Read the model definition and answer for the solid it produces. Units are mm, in the model's axes. Face numbers are marked on the shaded views. A direction names the side the tool comes from. Coordinates: 2 decimals unless noted, no trailing zeros. Order: outer loops, then holes, each group sorted by start corner. A loop starts at its lowest first (then second) coordinate and runs counter-clockwise, first axis right, second up. Notation, with made-up numbers: M -10,13.25 L 17,13.25 A15 ccw 17,33.25 Z; hole C 31.25,-22.5 d8. An arc over 180 degrees is marked long. Put each result on its own line as item: value.
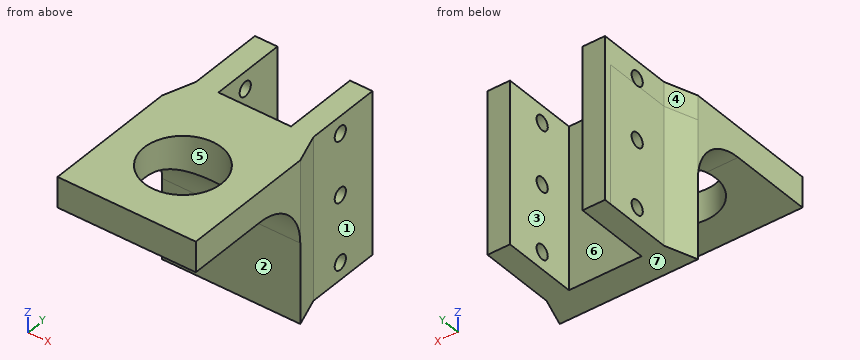
Autodesk Inventor part; units mm, degrees
ref_plane "YZ Plane" through (0, 0, 0) normal (1, 0, 0) x (0, 1, 0)
ref_plane "XZ Plane" through (0, 0, 0) normal (0, 1, 0) x (-1, 0, 0)
ref_plane "XY Plane" through (0, 0, 0) normal (0, 0, 1) x (1, 0, 0)
sketch "Sketch1" plane through (0, 0, 0) normal (0, 0, 1) x (1, 0, 0)
  line L0 (-25.4, -35.56) -> (25.4, -35.56)
  line L1 (25.4, -35.56) -> (25.4, 13.97)
  line L2 (25.4, 13.97) -> (-25.4, 13.97)
  line L3 (-25.4, 13.97) -> (-25.4, -35.56)
  line L4 (-25.4, -35.56) -> (25.4, 13.97) construction
  line L5 (25.4, -35.56) -> (-25.4, 13.97) construction
  line L6 (0, 25.146) -> (-12.7, 25.146)
  line L7 (-12.7, 25.146) -> (12.7, 25.146)
  line L8 (-12.7, 25.146) -> (-25.4, 13.97)
  line L9 (12.7, 25.146) -> (25.4, 13.97)
  line L10 (-12.7, 25.146) -> (-21.59, 25.146)
  line L11 (-21.59, 25.146) -> (-21.59, 50.546)
  line L12 (-21.59, 50.546) -> (-12.7, 50.546)
  line L13 (-12.7, 50.546) -> (-12.7, 25.146)
  line L14 (-21.59, 25.146) -> (-25.4, 13.97)
  line L15 (12.7, 25.146) -> (12.7, 50.546)
  line L16 (12.7, 50.546) -> (21.59, 50.546)
  line L17 (21.59, 50.546) -> (21.59, 25.146)
  line L18 (21.59, 25.146) -> (25.4, 13.97)
  line L19 (12.7, 25.146) -> (21.59, 25.146)
  circle A0 centre (0, -8.89) radius 14.224
  point P0 (0, 0)
  dimension "d1" = 49.53
  dimension "d2" = 50.8
  dimension "d6" = 8.89
  dimension "d7" = 25.4
  dimension "d8" = 8.89
  dimension "d47" = 11.176
  dimension "d51" = 28.448
  dimension "d52" = 34.036
  dimension "d53" = 43.18
extrude "Extrusion1" add sketch "Sketch1" along normal blind 8.89
sketch "Sketch3" plane through (0, 0, 0) normal (0, 0, -1) x (-1, 0, 0)
  circle A0 centre (0, 0) radius 14.224
  line L0 (21.5903, 3.302) -> (-21.59, 3.302)
  line L1 (-21.59, 3.302) -> (-21.59, 25.146)
  line L2 (-21.59, 25.146) -> (21.5903, 25.146)
  line L3 (21.5903, 25.146) -> (21.5903, 3.302)
  circle A1 centre (0, 0) radius 14.224
  line L4 (21.5903, 3.302) -> (-21.59, 25.146) construction
  line L5 (-21.59, 3.302) -> (21.5903, 25.146) construction
  line L6 (-25.4, -35.56) -> (-25.4, 13.97)
  line L7 (25.4, 13.97) -> (25.4, -35.56)
  line L8 (25.4, -35.56) -> (-25.4, -35.56)
  line L9 (25.4, 13.97) -> (25.4, -35.56)
  line L10 (21.59, 25.146) -> (25.4, 13.97)
  line L11 (21.59, 50.546) -> (21.59, 25.146)
  line L12 (12.7, 50.546) -> (21.59, 50.546)
  line L13 (12.7, 25.146) -> (12.7, 50.546)
  line L14 (-12.7, 25.146) -> (12.7, 25.146)
  line L15 (-12.7, 50.546) -> (-12.7, 25.146)
  line L16 (-21.59, 50.546) -> (-12.7, 50.546)
  line L17 (-21.59, 25.146) -> (-21.59, 50.546)
  line L18 (-25.4, 13.97) -> (-21.59, 25.146)
  line L19 (-25.4, -35.56) -> (-25.4, 13.97)
  line L20 (25.4, 3.302) -> (21.5903, 3.302)
  line L21 (-25.4, 3.302) -> (-21.59, 3.302)
  line L22 (0, 14.224) -> (-25.4, 14.224)
  point P0 (0.0002, 14.224)
  point P1 (-25.4, 13.97)
  point P2 (-13.8354, 3.302)
  point P3 (13.8354, 3.302)
  dimension "d13" = 28.448
extrude "Extrusion3" add sketch "Sketch3" along normal blind 50.8 contours A0 L22 L1 L2 L3 L0 | L0 L1 L22 A0 | L3 L10 L7 L20 | L21 L6 L18 L22 L1 | L22 L18 L1 | L2 L13 L12 L11 | L17 L16 L15 L2
sketch "Sketch5" plane through (21.59, 50.546, 8.89) normal (1, 0, 0) x (0, 0, -1)
  line L0 (59.69, -25.4) -> (59.69, 0)
  line L1 (0, -23.5788) -> (57.5469, -23.5788)
  line L2 (57.5469, 0) -> (57.5469, -23.5788)
  line L3 (59.69, 0) -> (59.69, -25.4)
  line L4 (59.69, 0) -> (0, 0)
  line L5 (0, -25.4) -> (0, 0)
  line L6 (59.69, -25.4) -> (0, -25.4)
  line L7 (0, -25.4) -> (0, -12.7)
  line L8 (0, -12.7) -> (57.5469, -12.7)
  circle A0 centre (6.35, -12.7) radius 2.6543
  circle A1 centre (53.34, -12.7) radius 2.6543
  circle A2 centre (28.7734, -12.7) radius 2.6543
  point P0 (8.89, -50.546)
  point P1 (59.69, -25.4)
  point P2 (31.4277, -12.7)
  point P3 (26.1191, -12.7)
  point P4 (55.9943, -12.7)
  point P5 (50.6857, -12.7)
  point P6 (9.0043, -12.7)
  point P7 (3.6957, -12.7)
  dimension "d39" = 12.7
  dimension "d40" = 5.3086
  dimension "d41" = 6.35
  dimension "d42" = 5.3086
  dimension "d43" = 6.35
  dimension "d44" = 5.3086
  dimension "d46" = 0
extrude "Extrusion4" cut sketch "Sketch5" against normal up to surface (43.18 mm away) contours A1 L8 | L8 A1 | A0 L8 | L8 A0 | A2 L8 | L8 A2
sketch "Sketch9" plane through (0, 0, -50.8) normal (0, 0, -1) x (-1, 0, 0)
  line L0 (-21.59, 50.546) -> (-12.7, 50.546)
  line L1 (13.335, -0.254) -> (-13.335, -0.254)
  line L2 (-13.335, -0.254) -> (-13.335, 50.546)
  line L3 (-13.335, 50.546) -> (13.335, 50.546)
  line L4 (13.335, 50.546) -> (13.335, -0.254)
  line L5 (-12.7, 25.146) -> (12.7, 25.146)
  line L6 (13.335, -0.254) -> (-13.335, 50.546) construction
  line L7 (-13.335, -0.254) -> (13.335, 50.546) construction
  line L8 (-25.4, -35.56) -> (-25.4, 13.97)
  line L9 (25.4, -13.97) -> (-25.4, -13.97)
  line L10 (-25.4, -13.97) -> (-25.4, 13.97)
  line L11 (-25.4, 13.97) -> (25.4, 13.97)
  line L12 (25.4, 13.97) -> (25.4, -13.97)
  line L13 (25.4, -13.97) -> (-25.4, 13.97) construction
  line L14 (-25.4, -13.97) -> (25.4, 13.97) construction
  point P0 (0, 0)
  point P1 (0, 25.146)
  point P2 (-13.335, 13.97)
  point P3 (13.335, 13.97)
  point P4 (-12.7, 50.546)
  dimension "d27" = 26.67
extrude "Extrusion5" cut sketch "Sketch9" against normal blind 42.8625
sketch "Sketch11" plane through (0, 0, 0) normal (0, 0, -1) x (-1, 0, 0)
  line L0 (25.4, 3.302) -> (13.8354, 3.302)
  line L1 (-13.8354, 3.302) -> (-25.4, 3.302)
  line L2 (-25.4, -35.56) -> (-25.4, 3.302)
  line L3 (25.4, -35.56) -> (-25.4, -35.56)
  line L4 (25.4, 3.302) -> (25.4, -35.56)
  line L5 (12.7, 25.146) -> (12.7, 50.546)
  line L6 (-12.7, 25.146) -> (12.7, 25.146)
  line L7 (-12.7, 50.546) -> (-12.7, 25.146)
  line L8 (-13.335, 50.546) -> (-12.7, 50.546)
  line L9 (-13.335, 13.97) -> (-13.335, 50.546)
  line L10 (-25.4, 13.97) -> (-13.335, 13.97)
  line L11 (-25.4, 3.302) -> (-25.4, 13.97)
  line L12 (-13.8354, 3.302) -> (-25.4, 3.302)
  arc A0 (13.8354, 3.302) -> (-13.8354, 3.302) centre (0, 0) ccw
  line L13 (25.4, 3.302) -> (13.8354, 3.302)
  line L14 (25.4, 13.97) -> (25.4, 3.302)
  line L15 (13.335, 13.97) -> (25.4, 13.97)
  line L16 (13.335, 50.546) -> (13.335, 13.97)
  line L17 (12.7, 50.546) -> (13.335, 50.546)
  arc A1 (13.8354, 3.302) -> (-13.8354, 3.302) centre (0, 0) ccw
extrude "Extrusion6" add sketch "Sketch11" along normal blind 2.286 contours L4 L3 L2 L1 A0 L0
sketch "Sketch12" plane through (0, 0, -7.9375) normal (0, 0, -1) x (-1, 0, 0)
  line L0 (12.7, 25.146) -> (12.7, 50.546)
  line L1 (-12.7, 25.146) -> (12.7, 25.146)
  line L2 (-12.7, 50.546) -> (-12.7, 25.146)
  line L3 (-13.335, 50.546) -> (-12.7, 50.546)
  line L4 (-13.335, 13.97) -> (-13.335, 50.546)
  line L5 (-25.4, 13.97) -> (-13.335, 13.97)
  line L6 (-25.4, 3.302) -> (-25.4, 13.97)
  line L7 (-13.8354, 3.302) -> (-25.4, 3.302)
  arc A0 (13.8354, 3.302) -> (-13.8354, 3.302) centre (0, 0) ccw
  line L8 (25.4, 3.302) -> (13.8354, 3.302)
  line L9 (25.4, 13.97) -> (25.4, 3.302)
  line L10 (13.335, 13.97) -> (25.4, 13.97)
  line L11 (13.335, 50.546) -> (13.335, 13.97)
  line L12 (12.7, 50.546) -> (13.335, 50.546)
extrude "Extrusion7" cut sketch "Sketch12" against normal blind 5.6515
sketch "Sketch13" plane through (0, 0, -2.286) normal (0, 0, -1) x (-1, 0, 0)
  line L0 (-12.7, 25.146) -> (12.7, 25.146)
  line L1 (-13.335, 13.97) -> (-13.335, 50.546)
  line L2 (12.7, 25.146) -> (-13.335, 25.146)
  line L3 (-13.335, 25.146) -> (-13.335, 50.546)
  line L4 (-13.335, 50.546) -> (12.7, 50.546)
  line L5 (12.7, 50.546) -> (12.7, 25.146)
  line L6 (13.335, 50.546) -> (13.335, 13.97)
  line L7 (12.7, 50.546) -> (13.335, 50.546)
  line L8 (13.335, 50.546) -> (13.335, 25.146)
  line L9 (13.335, 25.146) -> (12.7, 25.146)
  line L10 (12.7, 25.146) -> (12.7, 50.546)
  point P0 (0, 0)
  point P1 (-13.335, 25.146)
extrude "Extrusion8" cut sketch "Sketch13" against normal blind 37.211
sketch "Sketch14" plane through (0, 0, -2.286) normal (0, 0, -1) x (-1, 0, 0)
  circle A0 centre (0, 0) radius 14.224
  line L0 (25.4, 13.97) -> (25.4, -35.56)
  line L1 (13.335, 25.146) -> (-13.335, 25.146)
  line L2 (-13.335, 13.97) -> (-13.335, 25.146)
  line L3 (-25.4, 13.97) -> (-13.335, 13.97)
  line L4 (-25.4, -35.56) -> (-25.4, 13.97)
  line L5 (-25.4, -35.56) -> (25.4, -35.56)
  line L6 (25.4, 13.97) -> (25.4, -35.56)
  line L7 (13.335, 13.97) -> (25.4, 13.97)
  line L8 (13.335, 25.146) -> (13.335, 13.97)
  line L9 (-13.335, 13.97) -> (-13.335, 50.546)
  line L10 (-13.335, 50.546) -> (-21.59, 50.546)
  line L11 (-21.59, 50.546) -> (-21.59, 25.146)
  line L12 (-21.59, 25.146) -> (-25.4, 13.97)
  line L13 (-25.4, 13.97) -> (-13.335, 13.97)
  line L14 (13.335, 50.546) -> (13.335, 13.97)
  line L15 (13.335, 13.97) -> (25.4, 13.97)
  line L16 (25.4, 13.97) -> (21.59, 25.146)
  line L17 (21.59, 25.146) -> (21.59, 50.546)
  line L18 (21.59, 50.546) -> (13.335, 50.546)
  line L19 (-21.59, 25.146) -> (21.59, 25.146)
  line L20 (-25.4, 15.2659) -> (25.4, 15.2659)
  point P0 (25.4, 14.224)
  point P1 (25.4, 13.97)
  point P2 (-25.4, 13.97)
  point P3 (25.4, 13.97)
  point P4 (24.9582, 15.2659)
  point P5 (13.335, 15.2659)
  point P6 (-13.335, 15.2659)
  point P7 (-24.9582, 15.2659)
extrude "Extrusion9" add sketch "Sketch14" along normal up to surface (48.514 mm away) contours L20 L8 L19 L16 | L20 L2 L1 L8 | L20 L12 L19 L2
sketch "Sketch15" plane through (0, -8.89, 0) normal (0, 0, 1) x (1, 0, 0)
  circle A0 centre (0, 0) radius 14.224
  point P0 (0, 8.89)
extrude "Extrusion10" cut sketch "Sketch15" against normal blind 33.9725
sketch "Sketch16" plane through (-21.59, 50.546, 8.89) normal (0, 1, 0) x (1, 0, 0)
  line L0 (8.255, 0) -> (8.255, 59.69)
  line L1 (0, 59.69) -> (8.255, 59.69)
  line L2 (0, 59.69) -> (0, 0)
  line L3 (8.255, 0) -> (0, 0)
  line L4 (34.925, 59.69) -> (34.925, 0)
  line L5 (43.18, 0) -> (34.925, 0)
  line L6 (43.18, 59.69) -> (43.18, 0)
  line L7 (34.925, 59.69) -> (43.18, 59.69)
  point P0 (21.59, 8.89)
extrude "Extrusion11" add sketch "Sketch16" along normal blind 2.54
sketch "Sketch17" plane through (0, 0, -2.286) normal (0, 0, -1) x (-1, 0, 0)
  line L0 (-25.4, 13.97) -> (-13.335, 13.97)
  line L1 (13.335, 15.2659) -> (13.335, 13.97)
  line L2 (-13.335, 13.97) -> (13.335, 13.97)
  line L3 (13.335, 13.97) -> (13.335, 15.2659)
  line L4 (13.335, 15.2659) -> (-13.335, 15.2659)
  line L5 (-13.335, 15.2659) -> (-13.335, 13.97)
  point P0 (0, 0)
extrude "Extrusion12" add sketch "Sketch17" along normal up to surface (48.514 mm away)
fillet "Fillet5" radius 19.05 1 edges at (0, 13.97, -2.286)
equation "\"d9\" = d6"
properties part number "CH-4_DiffBarSupport"
Q1. For a pull along Y with two mould halves and no side action, classify the marked faces 5, 6 and 7 as +Y half, -Y half, draft (parallel to the pull), parting line (faces both ways), or undercut.
Answers below:
face 5: undercut
face 6: +Y half
face 7: draft
Q2. Consider line 1 along Z through (x, y) = (20.5, 37.5); line 2 along Y through (x, z) = (-19, 2.54); line 3 along X through (y, z) = (27, 4) (3 decimals). Determine where each line is inside the solid, lowest interval first.
Answers below:
line 1: z = -50.8 to -47.08, -41.82 to -22.52, -17.25 to -0.09, 5.17 to 8.89
line 2: y = -35.56 to 35.19, 40.5 to 53.09
line 3: x = -21.59 to -13.335, 13.335 to 21.59
Q3. Find section A-A on z = 2.54. Write down the section's boundary in (x, y) (3 decimals), plus the area to 3 significant figures.
Answers below:
outline: M -25.4,-35.56 L 25.4,-35.56 L 25.4,13.97 L 21.59,25.146 L 21.59,35.192 L 13.335,35.192 L 13.335,25.146 L -13.335,25.146 L -13.335,35.192 L -21.59,35.192 L -21.59,25.146 L -25.4,13.97 Z; M -21.59,40.5 L -13.335,40.5 L -13.335,53.086 L -21.59,53.086 Z; M 13.335,40.5 L 21.59,40.5 L 21.59,53.086 L 13.335,53.086 Z; hole C 0,-8.89 d28.448
area: 2,780 mm^2
Q4. Find section C-C on y = -8.89. Write down the section's boundary in (x, z).
Answers below:
outline: M -25.4,-2.29 L -14.22,-2.29 L -14.22,8.89 L -25.4,8.89 Z; M 14.22,-2.29 L 25.4,-2.29 L 25.4,8.89 L 14.22,8.89 Z
Q5. Find section B-B on x = 0. Write down the section's boundary in (y, z).
Answers below:
outline: M -35.56,-2.29 L -23.11,-2.29 L -23.11,8.89 L -35.56,8.89 Z; M 5.33,-5.38 A19.05 cw 13.97,-21.34 L 13.97,-50.8 L 25.15,-50.8 L 25.15,8.89 L 5.33,8.89 Z
Q6. A tool of negligible diameter and unlimited length cuts with its end or side. For the marked faces 1, 2, 3 and 4, from which of +Z, -Z, +X, -X, +Y, -Y can it reach the whole face along a straight path? Write none if from no direction.
Answers below:
face 1: +Z, -Z, +X, +Y
face 2: -Z, +X, -X, -Y
face 3: +Z, -Z, +Y
face 4: +Z, -Z, -X, +Y
Q7. Given pin 1 (5 mm diameter, centred on y = 37.846, z = -44.45, fed in from -X); pin 2 (14 mm diameter, centred on y = 36, z = -19.5, fed in from +X); pin 3 (10 mm diameter, centred on x = 12.5, y = -25.5, fed in from -Z); pin 4 (20.5 mm diameter, centred on y = 37, z = -13.5, fed in from -X), each flat-ended and moving along its own axis, determine where each tip first touches the part or whether it passes through.
Answers below:
pin 1: passes through
pin 2: stops at x = 21.59
pin 3: stops at z = -2.29
pin 4: stops at x = -21.59
Q8. Find section D-D on z = -20. Write down the section's boundary in (x, y) (3 decimals), plus the area to 3 significant figures.
Answers below:
outline: M -25.4,13.923 L 25.4,13.923 L 25.4,13.97 L 21.59,25.146 L 21.59,35.194 L 13.335,35.194 L 13.335,25.146 L -13.335,25.146 L -13.335,35.194 L -21.59,35.194 L -21.59,25.146 L -25.4,13.97 Z; M -21.59,40.498 L -13.335,40.498 L -13.335,53.086 L -21.59,53.086 L -21.59,50.546 Z; M 13.335,40.498 L 21.59,40.498 L 21.59,53.086 L 13.335,53.086 Z
area: 901 mm^2
